Can you work these out from the model? Positions are in its coordinate system, mm. A direction names the side the tool comes from. Round coordinates to 2 decimals unless told otherwise and drop trailing zeros. Order: outer loops, then holes, each group sorted by start corner. A loop starts at its lowest first (then second) coordinate and runs counter-clockwise, first axis right, second up.
Q1. For faces 4 (the face through (-11, -103.3, 55)), 5 (the face through (20.68, -142.33, 81.13)), which set-ups out of +Z, -Z, +X, -X, +Y, -Y let a thin tool reach every point of the face, with its end or its side?
Q2. We'd pull the mould along X, two halves only. Please class faces 1 (the face through (-59.17, -123.57, 35.21)), 2 (the face through (39.1, -118.6, 35.4)), 3 (the face through (13.085, -142.328, 68.281)): pulls with the +X half, pulls with the -X half, needs draft (parallel to the pull), parting line crosses it, or undercut.
Q3. If we section it at C-C (z = 59.5): Please give me the cut outline in (x, y).
Q4. Will these pins go through, and if not, where does the flat tip stop? P1, Ø1.5, axis at x = 11.5, y = -126, coming from the +Z side; P2, Ø12, axis at y = -112.5, z = 39, coming from the -X side.
Q5. If we section it at D-D (z = 69): Please give me the cut outline in (x, y), plus the area to 3 significant figures.
Q6. If we section it at A-A (x = -17.5): Please give me the cut outline in (y, z), plus the area to 3 significant figures.
Q7. If we section it at B-B (y = -114.3): Please give me the cut outline in (x, z).
Q8. If I drill on line 1 (Y direction, x = -38.5, z = 53); line 2 (X direction, y = -141, z = 72); line 3 (X direction, y = -141.15, z = 72.9), over which ranges is the centre line in solid material (lowest first)?
from build123d import *

# Parameters (mm, degrees)
SKETCH1_R               = 5
BOSS_EXTRUDE1_DEPTH     = 50
SKETCH2_R               = 5
CUT_EXTRUDE1_DEPTH      = 112.791815443
CUT_EXTRUDE2_DEPTH      = 177.903545314
CUT_EXTRUDE2_DEPTH_BACK = 177.903545314
SKETCH3_W               = 65.68648631
SKETCH3_H               = 37


with BuildPart() as part:
    # Sketch1 → Boss-Extrude1 (new body)
    with BuildSketch(Plane.XY.offset(32.9)):
        Polygon((-40, -144.299876296), (40, -144.299876296), (40, -99.299876296), (-40, -99.299876296), (-60, -99.299876296), (-60, -144.299876296), align=None)
        with Locations((17.5, -114.3)):
            Circle(SKETCH1_R, mode=Mode.SUBTRACT)
        with Locations((-17.5, -114.3)):
            Circle(SKETCH1_R, mode=Mode.SUBTRACT)
    extrude(amount=BOSS_EXTRUDE1_DEPTH)

    # Sketch2 → Cut-Extrude1 (cut, through all)
    with BuildSketch(Plane.XZ.offset(144.299876296)):
        with BuildLine():
            Line((-60, 82.9), (-60, 32.9))
            Line((-60, 32.9), (-44.410826478, 76.281766549))
            ThreePointArc((-44.410826478, 76.281766549), (-40.752492265, 81.07978195), (-35, 82.9))
            Line((-35, 82.9), (-60, 82.9))
        make_face()
        with BuildLine():
            Line((24.410826478, 76.281766549), (40, 32.9))
            Line((40, 32.9), (40, 82.9))
            Line((40, 82.9), (15, 82.9))
            ThreePointArc((15, 82.9), (20.752492265, 81.07978195), (24.410826478, 76.281766549))
        make_face()
        with Locations(Location((15, 72.9, 0), (0, 0, 270))):
            Circle(SKETCH2_R)
        with Locations(Location((-35, 72.9, 0), (0, 0, 270))):
            Circle(SKETCH2_R)
    extrude(amount=-CUT_EXTRUDE1_DEPTH, mode=Mode.SUBTRACT)

    # Sketch3 → Cut-Extrude2 (cut, two sides: drawn at the far end of the back side and taken through both)
    with BuildSketch(Plane(origin=(0, 0, 0), x_dir=(0, 0, -1), z_dir=(1, 0, 0)).offset(-CUT_EXTRUDE2_DEPTH_BACK)):
        with Locations((-69.743243155, -121.799876296)):
            Rectangle(SKETCH3_W, SKETCH3_H)
    extrude(amount=CUT_EXTRUDE2_DEPTH + CUT_EXTRUDE2_DEPTH_BACK, mode=Mode.SUBTRACT)


solid = part.part
Solution:
1. face 4: +Z, +X, -X
1. face 5: +Z, +X, +Y, -Y
2. face 1: pulls with the -X half
2. face 2: pulls with the +X half
2. face 3: undercut
3. outline: (-50.44, -144.3) - (30.44, -144.3) - (30.44, -140.3) - (-50.44, -140.3) - close; (-50.44, -103.3) - (30.44, -103.3) - (30.44, -99.3) - (-50.44, -99.3) - close
4. P1: stops at z = 36.9
4. P2: stops at x = -59.96
5. outline: (-47.03, -144.3) - (-38.13, -144.3) - (-38.13, -140.3) - (-47.03, -140.3) - close; (-47.03, -103.3) - (-38.13, -103.3) - (-38.13, -99.3) - (-47.03, -99.3) - close; (-31.87, -144.3) - (11.87, -144.3) - (11.87, -140.3) - (-31.87, -140.3) - close; (-31.87, -103.3) - (11.87, -103.3) - (11.87, -99.3) - (-31.87, -99.3) - close; (18.13, -144.3) - (27.03, -144.3) - (27.03, -140.3) - (18.13, -140.3) - close; (18.13, -103.3) - (27.03, -103.3) - (27.03, -99.3) - (18.13, -99.3) - close
5. area: 492 mm2
6. outline: (-144.3, 32.9) - (-119.3, 32.9) - (-119.3, 36.9) - (-140.3, 36.9) - (-140.3, 82.9) - (-144.3, 82.9) - close; (-109.3, 32.9) - (-99.3, 32.9) - (-99.3, 82.9) - (-103.3, 82.9) - (-103.3, 36.9) - (-109.3, 36.9) - close
6. area: 508 mm2
7. outline: (-60, 32.9) - (-22.5, 32.9) - (-22.5, 36.9) - (-58.56, 36.9) - close; (-12.5, 32.9) - (12.5, 32.9) - (12.5, 36.9) - (-12.5, 36.9) - close; (22.5, 32.9) - (40, 32.9) - (38.56, 36.9) - (22.5, 36.9) - close
8. line 1: y = -144.3 to -140.3, -103.3 to -99.3
8. line 2: x = -45.95 to -39.92, -30.08 to 10.08, 19.92 to 25.95
8. line 3: x = -45.63 to -40, -30 to 10, 20 to 25.63
